Geometry check sheet. Reference: the model listing, model coordinates, mm. Round coordinates to 2 decimals unless told otherwise and drop trailing zeros. Loops run counter-clockwise (first coordinate to the right, second up) from the corner with the lowest first, then second, coordinate; pieces in that order, holes last. Notation, with made-up numbers: (40, 4) - (52, 4) arc R27 cw to (52, 43) - close; hole circle Ø10 at (88, -22.5). An arc over 180 degrees is marked (long way). Answer as CSV lines item,"result". Start each with the question number.
1) Cross-section at C-C on z = 14. Record the boundary of the cut face in (x, y).
2) Cross-section at B-B on y = -0.7. Record the boundary of the cut face in (x, z).
3) Thickness scan on line 1 along X through (y, z) = (-0.1, 15); line 2 along X through (y, z) = (-0.7, -14); line 3 along X through (y, z) = (0.95, 13). Record the ranges inside material, lowest first.
4) Cross-section at D-D on x = 0. Record the boundary of the cut face in (y, z), and give its area (3 significant figures).
5) Cross-section at A-A on z = -16. Record the boundary of the cut face in (x, y), and give its area (3 significant figures).
6) Depth check by flat-ended pin: P1, Ø6.5, axis at x = -15.897, z = 15.892, coming from the +Y side; P2, Ø3, axis at x = -11.5, z = -13.5, coming from the -Y side. Enter the tip coordinate at first touch or a pass-through.
from build123d import *

# Parameters (mm, degrees)
F0_R     = 4
F1_DEPTH = 1.5


with BuildPart() as f1:
    # F0 (on Front) → F1 (new body, symmetric)
    with BuildSketch(Plane.XZ):
        with BuildLine():
            Line((-64.897, 24.892), (-64.897, -24.892))
            Line((-64.897, -24.892), (-17, -24.892))
            ThreePointArc((-17, -24.892), (0, -7.892), (17, -24.892))
            Line((17, -24.892), (64.897, -24.892))
            Line((64.897, -24.892), (64.897, 24.892))
            Line((64.897, 24.892), (-64.897, 24.892))
        make_face()
        with Locations((-15.897, 15.892)):
            Circle(F0_R, mode=Mode.SUBTRACT)
        with Locations((17.103, 15.892)):
            Circle(F0_R, mode=Mode.SUBTRACT)
    extrude(amount=F1_DEPTH, both=True)


solid = f1.part
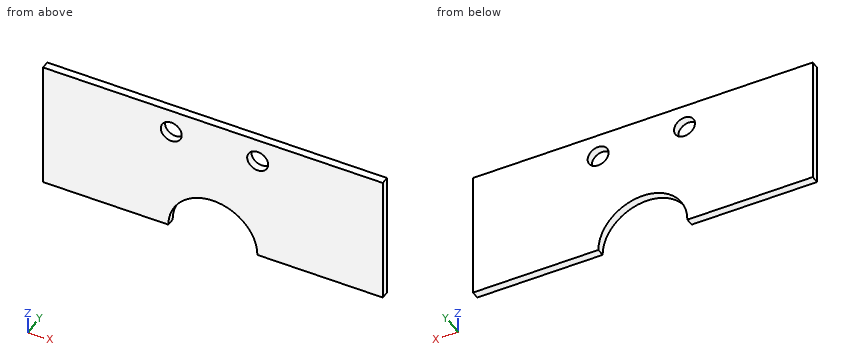
Answer block:
1,outline,"(-64.9, -1.5) - (-19.42, -1.5) - (-19.42, 1.5) - (-64.9, 1.5) - close; (-12.37, -1.5) - (13.58, -1.5) - (13.58, 1.5) - (-12.37, 1.5) - close; (20.63, -1.5) - (64.9, -1.5) - (64.9, 1.5) - (20.63, 1.5) - close"
2,outline,"(-64.9, -24.89) - (-17, -24.89) arc R17 cw to (17, -24.89) - (64.9, -24.89) - (64.9, 24.89) - (-64.9, 24.89) - close; hole circle Ø8 at (-15.9, 15.89); hole circle Ø8 at (17.1, 15.89)"
3,line 1,"x = -64.9 to -19.8, -12 to 13.2, 21 to 64.9"
3,line 2,"x = -64.9 to -13.05, 13.05 to 64.9"
3,line 3,"x = -64.9 to -18.66, -13.13 to 14.34, 19.87 to 64.9"
4,outline,"(-1.5, -7.89) - (1.5, -7.89) - (1.5, 24.89) - (-1.5, 24.89) - close"
4,area,"98.4 mm^2"
5,outline,"(-64.9, -1.5) - (-14.49, -1.5) - (-14.49, 1.5) - (-64.9, 1.5) - close; (14.49, -1.5) - (64.9, -1.5) - (64.9, 1.5) - (14.49, 1.5) - close"
5,area,"302 mm^2"
6,P1,"passes through"
6,P2,"stops at y = -1.5"
